from build123d import *

# Parameters (mm, degrees)
BOSS_EXTRUDE1_DEPTH = 5
BOSS_EXTRUDE2_DEPTH = 31.75
FILLET1_R           = 5


with BuildPart() as part:
    # Sketch1 → Boss-Extrude1 (new body)
    with BuildSketch(Plane.XY):
        Polygon((-44.432958232964275, 15.875000000000018), (44.46704176703572, 15.875000000000021), (44.467041767035624, -15.874999999999979), (-44.43295823296417, -15.875000000000448), (-53.51922912646058, -13.017500000000476), align=None)
    extrude(amount=BOSS_EXTRUDE1_DEPTH)

    # Sketch2 → Boss-Extrude2 (add)
    with BuildSketch(Plane(origin=(0, 0, 0), x_dir=(-1, 0, 0), z_dir=(0, 0, -1))):
        Polygon((-39.467041767035624, 15.875000000000021), (-39.467041767035624, -15.875000000000448), (-44.467041767035624, -15.874999999999979), (-44.46704176703572, 15.875000000000021), align=None)
        Polygon((48.749533119375855, -14.51750000000046), (39.191534049354715, 15.875000000000021), (44.432958232964275, 15.875000000000018), (53.51922912646058, -13.017500000000476), align=None)
    extrude(amount=BOSS_EXTRUDE2_DEPTH)

    # Fillet1
    fillet1_edges = [part.edges().sort_by_distance(p)[0] for p in [
        (-48.97609367971243, 1.4287499999997717, 5),
        (-43.970533584365285, 0.6787499999997806, 0),
        (39.467041767035624, -2.1316e-13, 0),
        (44.46704176703567, 2.132e-14, 5),
    ]]
    fillet(fillet1_edges, radius=FILLET1_R)


solid = part.part
Design review of the part built by this model. Coordinates are the model's own, in mm. A direction names the side the tool comes from. Round coordinates to 2 decimals unless told otherwise and drop trailing zeros. Loops run counter-clockwise (first coordinate to the right, second up) from the corner with the lowest first, then second, coordinate; pieces in that order, holes last. Notation, with made-up numbers: (3, -37.75) - (48, -37.75) arc R19 cw to (48, -5.75) - close; hole circle Ø3 at (24, 0). An arc over 180 degrees is marked (long way). One line per item, written item: value. Start each with the question number.
1) For faces 1 (the flat face through (39.467, 0, -18)), 2 (the flat face through (-44.037, 0.466, -18.188)), 3 (the flat face through (-49.04, 1.23, -16.1)), list the 3-axis set-ups (+Z, -Z, +X, -X, +Y, -Y) from which the entire face can be reached by the end or side of a thin tool; tool diameter is ignored.
2) Consider section A-A on z = -27. Give the boundary of the cut face in (x, y) (1 decimal), then the cut area to 3 significant figures.
3) To check wall thickness, follow L1, parallel to Z at x = -25.5, y = -11.5; L2, parallel to X at y = -3, z = -16; L3, parallel to X at y = 9, z = -27. State the ranges of each line that lie inside material, in increasing order. Write a range as from..to.
4) Draft analysis for pull direction X (two halves, no side actions). For faces 4 (the cylindrical face through (-47.239, 1.94, 3.574)), 5 (the flat face through (6.4, -15.875, 0.3)), 6 (the cylindrical face through (-42.3, 1.22, -1.5)), state which applies: +X half, -X half, draft (parallel to the pull), parting line (faces both ways), or undercut.
5) Consider section B-B on x = -13.5. Give the boundary of the cut face in (y, z) (3 decimals), then the cut area to 3 significant figures.
6) Insertion check: pin 1 Ø16 at (x, y) = (-7.5, 4) entering from -Z; pin 2 Ø8 at (y, z) = (10.5, -0.5) entering from -X; pin 3 Ø10 at (y, z) = (-2, -26.5) entering from -X. Each pin has a flat end and moves straight along its axis. Give the tip position at first contact, or say it passes through.
Reported:
1. face 1: -Z, +Y, -Y
1. face 2: -Z, -Y
1. face 3: +Z, -Z, -X, +Y
2. outline: (-53.5, -13) - (-48.7, -14.5) - (-39.2, 15.9) - (-44.4, 15.9) - close; (39.5, -15.9) - (44.5, -15.9) - (44.5, 15.9) - (39.5, 15.9) - close
2. area: 314 mm^2
3. L1: z = 0..5
3. L2: x = -50.37..-45.13, 39.47..44.47
3. L3: x = -46.6..-41.35, 39.47..44.47
4. face 4: -X half
4. face 5: draft
4. face 6: undercut
5. outline: (-15.875, 0) - (15.875, 0) - (15.875, 5) - (-15.875, 5) - close
5. area: 159 mm^2
6. pin 1: stops at z = 0
6. pin 2: stops at x = -47.38
6. pin 3: stops at x = -51.63
